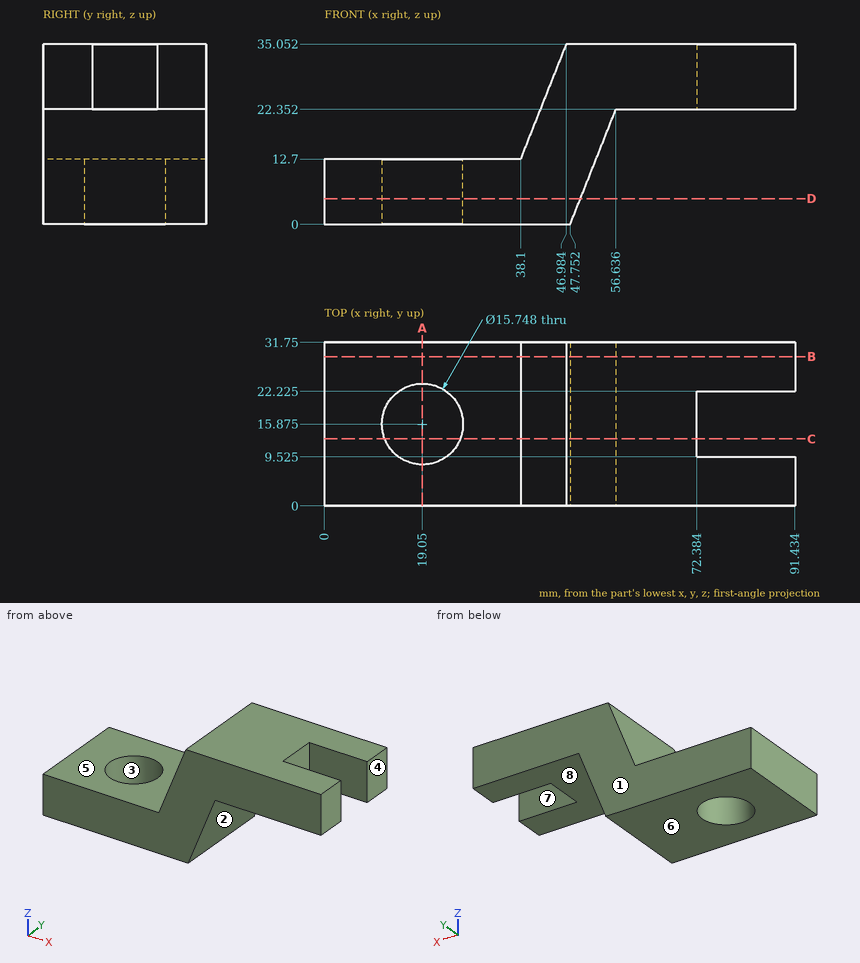
Part print with two shaded views. Sizes in mm from the minimum x, y, z corner. A direction names the side the tool comes from. Coordinates: 2 decimals unless noted, no trailing zeros. Write each loop counter-clockwise with the first axis right and the second up, starting at its lowest first coordinate (ties: lowest second). Pieces come first, ordered by that corner, then holes. Notation, with made-up numbers: (-18.5, -40) -> (36.5, -40) arc R14 cw to (36.5, -32) -> close; hole circle Ø1 at (79.5, 19.25). An arc over 180 degrees is marked (long way). Return JSON: item names as keys, results as strings. Group by question number.
Q1. Pull direction X, two halves, no side cores. Call the marked faces 1, 2 and 3: released by +X, released by -X, zero draft, split by the parting line, or undercut.
Q2. Drill centre lines: line 1 (Y direction, x = 19.05, z = 2.5); line 2 (Y direction, x = 82, z = 26) (3 decimals); line 3 (Z direction, x = 58.5, y = 2). Where is each one in solid material? Low to high.
Q3. Cut at B-B, the plane y = 29. Give the cut face in (x, z).
Q4. Cut at A-A, the plane x = 19.05. Give the cut face in (y, z), then the cut area to 3 significant figures.
Q5. Flat gauge pins, fed straight in: pin 1 (5 mm diameter, centred on y = 24, z = 5, fed in from +X); pin 2 (1 mm diameter, centred on x = 65.5, y = 9, fed in from -Z); pin 3 (3 mm diameter, centred on y = 26, z = 29.5, fed in from -X). Where does each tip first touch, or does it go through?
Q6. Cut at D-D, the plane z = 5. Give the cut face in (x, y) (3 decimals), then the cut area to 3 significant figures.
Q7. Which spindle directions (+Z, -Z, +X, -X, +Y, -Y) get a long thin tool onto all of the face, cutting with end or side? Do the marked faces 4, 5, 6, 7 and 8. Say none if no direction does.
Q8. Cut at C-C, the plane y = 13. Give the cut face in (x, z).
Returned:
{
 "1": {"face 1": "zero draft", "face 2": "released by +X", "face 3": "undercut"},
 "2": {"line 1": "y = 0 to 8, 23.75 to 31.75", "line 2": "y = 0 to 9.525, 22.225 to 31.75", "line 3": "z = 22.35 to 35.05"},
 "3": {"outline": "(0, 0) -> (47.75, 0) -> (56.64, 22.35) -> (91.43, 22.35) -> (91.43, 35.05) -> (46.98, 35.05) -> (38.1, 12.7) -> (0, 12.7) -> close"},
 "4": {"outline": "(0, 0) -> (8, 0) -> (8, 12.7) -> (0, 12.7) -> close; (23.75, 0) -> (31.75, 0) -> (31.75, 12.7) -> (23.75, 12.7) -> close", "area": "203 mm2"},
 "5": {"pin 1": "stops at x = 50.73", "pin 2": "stops at z = 22.35", "pin 3": "stops at x = 44.18"},
 "6": {"outline": "(0, 0) -> (49.739, 0) -> (49.739, 31.75) -> (0, 31.75) -> close; hole circle Ø15.748 at (19.05, 15.875)", "area": "1,380 mm2"},
 "7": {"face 4": "+Z, -Z, +X, +Y, -Y", "face 5": "+Z, -X, +Y, -Y", "face 6": "-Z, +X, -X, +Y, -Y", "face 7": "+Z, -Z, +X", "face 8": "-Z, +X, +Y, -Y"},
 "8": {"outline": "(0, 0) -> (11.72, 0) -> (11.72, 12.7) -> (0, 12.7) -> close; (26.38, 0) -> (47.75, 0) -> (56.64, 22.35) -> (72.38, 22.35) -> (72.38, 35.05) -> (46.98, 35.05) -> (38.1, 12.7) -> (26.38, 12.7) -> close"}
}
